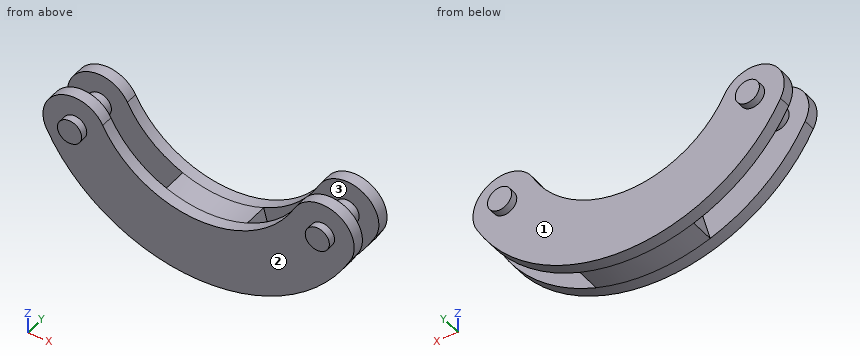
```python
from build123d import *

# Parameters (mm, degrees)
BOSS_EXTRUDE1_DEPTH = 9.5
BOSS_EXTRUDE2_DEPTH = 19
BOSS_EXTRUDE3_DEPTH = 9.5
SKETCH5_R           = 9.5
CUT_EXTRUDE1_DEPTH  = 154.110072724
BOSS_EXTRUDE4_START = 6
SKETCH5_2_R         = 9.5
BOSS_EXTRUDE4_DEPTH = 50


with BuildPart() as part:
    # Sketch2 → Boss-Extrude1 (new body)
    with BuildSketch(Plane(origin=(0, 0, 0), x_dir=(1, 0, 0), z_dir=(0, 1, 0))):
        with BuildLine():
            ThreePointArc((119.580217293, -46.896332496), (0, 25), (-119.580217293, -46.896332496))
            ThreePointArc((-119.580217293, -46.896332496), (-109.224504437, -80.701054226), (-75.419782707, -70.34534137))
            ThreePointArc((-75.419782707, -70.34534137), (0, -25), (75.419782707, -70.34534137))
            ThreePointArc((75.419782707, -70.34534137), (109.224504437, -80.701054226), (119.580217293, -46.896332496))
        make_face()
    extrude(amount=BOSS_EXTRUDE1_DEPTH)

    # Sketch3 → Boss-Extrude2 (add)
    with BuildSketch(Plane(origin=(0, 9.5, 0), x_dir=(1, 0, 0), z_dir=(0, 1, 0))):
        with BuildLine():
            Line((-44.843451744, 17.358040295), (-31.843255272, -31.159353446))
            ThreePointArc((-31.843255272, -31.159353446), (0, -25), (31.843255272, -31.159353446))
            Line((31.843255272, -31.159353446), (44.843451744, 17.358040295))
            ThreePointArc((44.843451744, 17.358040295), (0, 25), (-44.843451744, 17.358040295))
        make_face()
    extrude(amount=BOSS_EXTRUDE2_DEPTH)

    # Sketch4 → Boss-Extrude3 (add)
    with BuildSketch(Plane(origin=(0, 28.5, 0), x_dir=(1, 0, 0), z_dir=(0, 1, 0))):
        with BuildLine():
            ThreePointArc((119.580217293, -46.896332496), (0, 25), (-119.580217293, -46.896332496))
            ThreePointArc((-119.580217293, -46.896332496), (-109.224504437, -80.701054226), (-75.419782707, -70.34534137))
            ThreePointArc((-75.419782707, -70.34534137), (0, -25), (75.419782707, -70.34534137))
            ThreePointArc((75.419782707, -70.34534137), (109.224504437, -80.701054226), (119.580217293, -46.896332496))
        make_face()
    extrude(amount=BOSS_EXTRUDE3_DEPTH)

    # Sketch5 → Cut-Extrude1 (cut, through all)
    with BuildSketch(Plane(origin=(0, 38, 0), x_dir=(1, 0, 0), z_dir=(0, 1, 0))):
        with Locations(Location((-97.5, -58.620836933, 0), (0, 0, 270))):
            Circle(SKETCH5_R)
        with Locations(Location((97.5, -58.620836933, 0), (0, 0, 270))):
            Circle(SKETCH5_R)
    extrude(amount=-CUT_EXTRUDE1_DEPTH, mode=Mode.SUBTRACT)

    # Sketch5_2 → Boss-Extrude4 (add)
    with BuildSketch(Plane(origin=(0, 38, 0), x_dir=(1, 0, 0), z_dir=(0, 1, 0)).offset(BOSS_EXTRUDE4_START)):
        with Locations(Location((-97.5, -58.620836933, 0), (0, 0, 270))):
            Circle(SKETCH5_2_R)
        with Locations(Location((97.5, -58.620836933, 0), (0, 0, 270))):
            Circle(SKETCH5_2_R)
    extrude(amount=-BOSS_EXTRUDE4_DEPTH)


solid = part.part
```
For this review, take the finished solid that the model builds, in its own axes (mm). Face numbers are marked on the shaded views. Round coordinates to 2 decimals unless told otherwise and drop trailing zeros. Write each loop counter-clockwise with the first axis right and the second up, starting at its lowest first coordinate (ties: lowest second). Pieces come first, ordered by that corner, then holes. Notation, with made-up numbers: (1, -7) - (33, -7) arc R33 ccw to (33, 29) - close; hole circle Ø2 at (74.25, 75). An arc over 180 degrees is marked (long way). Answer as CSV lines item,"result". Start each with the question number.
(1) Add section B-B, the plane x = -65. State the section outline as (y, z) points, plus the area to 3 significant figures.
(2) For pin 1 (5 mm diameter, centred on x = 92.5, y = 7, fed in from +Z); pin 2 (12 mm diameter, centred on x = -13, y = 37, fed in from -Z); pin 3 (5 mm diameter, centred on x = -85.5, z = 23.5, fed in from +Y), all flat-tipped, find the tip position at first contact; note any pin that passes through.
(3) Mouldability with a two-part tool opening along Y and no side actions: class the marked faces 1, 2 and 3 as +Y half, -Y half, draft (parallel to the pull), parting line (faces both ways), or undercut.
(4) For line 1 (Y direction, x = -88, z = 22); line 2 (X direction, y = 19, z = 57.5); line 3 (X direction, y = 29, z = 58.5), list the stretches that pass through material, from the lowest coordinate up.
(5) Add section D-D, the plane x = 97.5. State the section outline as (y, z) points, plus the area to 3 significant figures.
(6) Add section C-C, the plane z = 5. State the section outline as (x, y) points.
(7) Add section A-A, the plane y = 13. State the section outline as (x, z) points.
From the geometry:
1,outline,"(0, -8.38) - (9.5, -8.38) - (9.5, 55.01) - (0, 55.01) - close; (28.5, -8.38) - (38, -8.38) - (38, 55.01) - (28.5, 55.01) - close"
1,area,"1,200 mm²"
2,pin 1,"stops at z = 83.5"
2,pin 2,"stops at z = -24.82"
2,pin 3,"stops at y = 38"
3,face 1,"+Y half"
3,face 2,"-Y half"
3,face 3,"undercut"
4,line 1,"y = 0 to 9.5, 28.5 to 38"
4,line 2,"x = -106.93 to -88.07, 88.07 to 106.93"
4,line 3,"x = -122.5 to -67.82, 67.82 to 122.5"
5,outline,"(-6, 49.12) - (0, 49.12) - (0, 16.45) - (9.5, 16.45) - (9.5, 49.12) - (28.5, 49.12) - (28.5, 16.45) - (38, 16.45) - (38, 49.12) - (44, 49.12) - (44, 68.12) - (38, 68.12) - (38, 83.62) - (28.5, 83.62) - (28.5, 68.12) - (9.5, 68.12) - (9.5, 83.62) - (0, 83.62) - (0, 68.12) - (-6, 68.12) - close"
5,area,"1,870 mm²"
6,outline,"(-84.99, 0) - (84.99, 0) - (84.99, 9.5) - (38.85, 9.5) - (38.85, 28.5) - (84.99, 28.5) - (84.99, 38) - (-84.99, 38) - (-84.99, 28.5) - (-38.85, 28.5) - (-38.85, 9.5) - (-84.99, 9.5) - close"
7,outline,"circle Ø19 at (-97.5, 58.62); (-44.84, -17.36) arc R135.39 ccw to (44.84, -17.36) - (31.84, 31.16) arc R85.39 cw to (-31.84, 31.16) - close; circle Ø19 at (97.5, 58.62)"
